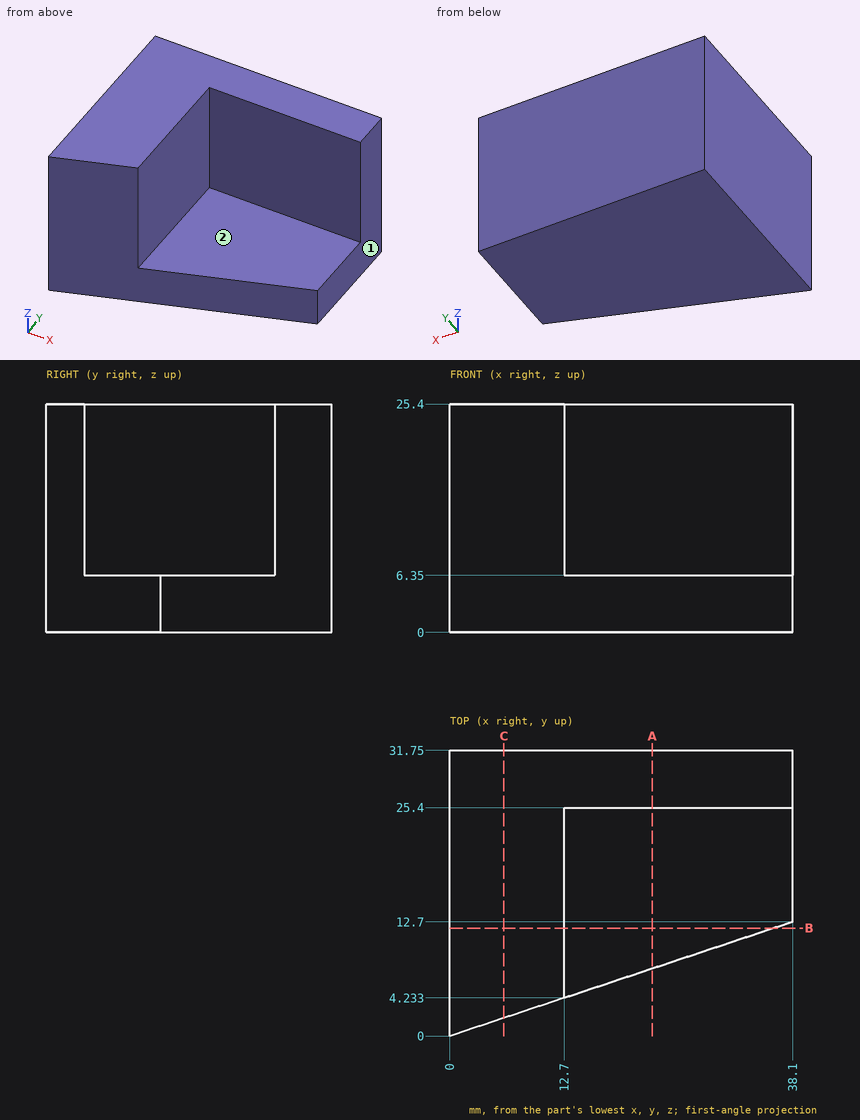
Could you check a few things on this drawing? It's one solid part, dimensions in mm from its lowest x, y, z. A direction names the side the tool comes from. Round coordinates to 2 decimals unless told otherwise and drop trailing zeros. Write each loop counter-clockwise with the first axis right and the second up, starting at its lowest first coordinate (ties: lowest second). Pieces come first, ordered by that corner, then holes.
Q1. If we section it at A-A on x = 22.5: Write out the boundary of the cut face in (y, z).
Q2. Will these pins go through, and if not, where does the flat tip stop? P1, Ø9.5, axis at x = 30.5, z = 18.5, coming from the -Y side; P2, Ø6.5, axis at x = 30.5, y = 13.5, coming from the +Z side; P3, Ø1.5, axis at x = 6.5, z = 15.5, coming from the -Y side.
Q3. If we section it at B-B on y = 12: Write out the boundary of the cut face in (x, z).
Q4. Please list where these lines run through material, in increasing order: probe 1 along Z at (x, y) = (25, 15); probe 2 along X at (y, z) = (12.5, 23.5); probe 3 along Y at (x, z) = (21, 13.75).
Q5. If we section it at C-C on x = 6: Write out the boundary of the cut face in (y, z), plus the area to 3 significant figures.
Q6. Which directions (+Z, -Z, +X, -X, +Y, -Y) give clear straight access to the entire face, cutting with the end or side of a thin tool? Please do the marked faces 1 and 2.
Answer below:
1. outline: (7.5, 0) - (31.75, 0) - (31.75, 25.4) - (25.4, 25.4) - (25.4, 6.35) - (7.5, 6.35) - close
2. P1: stops at y = 25.4
2. P2: stops at z = 6.35
2. P3: stops at y = 1.92
3. outline: (0, 0) - (36, 0) - (36, 6.35) - (12.7, 6.35) - (12.7, 25.4) - (0, 25.4) - close
4. probe 1: z = 0 to 6.35
4. probe 2: x = 0 to 12.7
4. probe 3: y = 25.4 to 31.75
5. outline: (2, 0) - (31.75, 0) - (31.75, 25.4) - (2, 25.4) - close
5. area: 756 mm2
6. face 1: +Z, -Z, +X, +Y, -Y
6. face 2: +Z, +X, -Y
